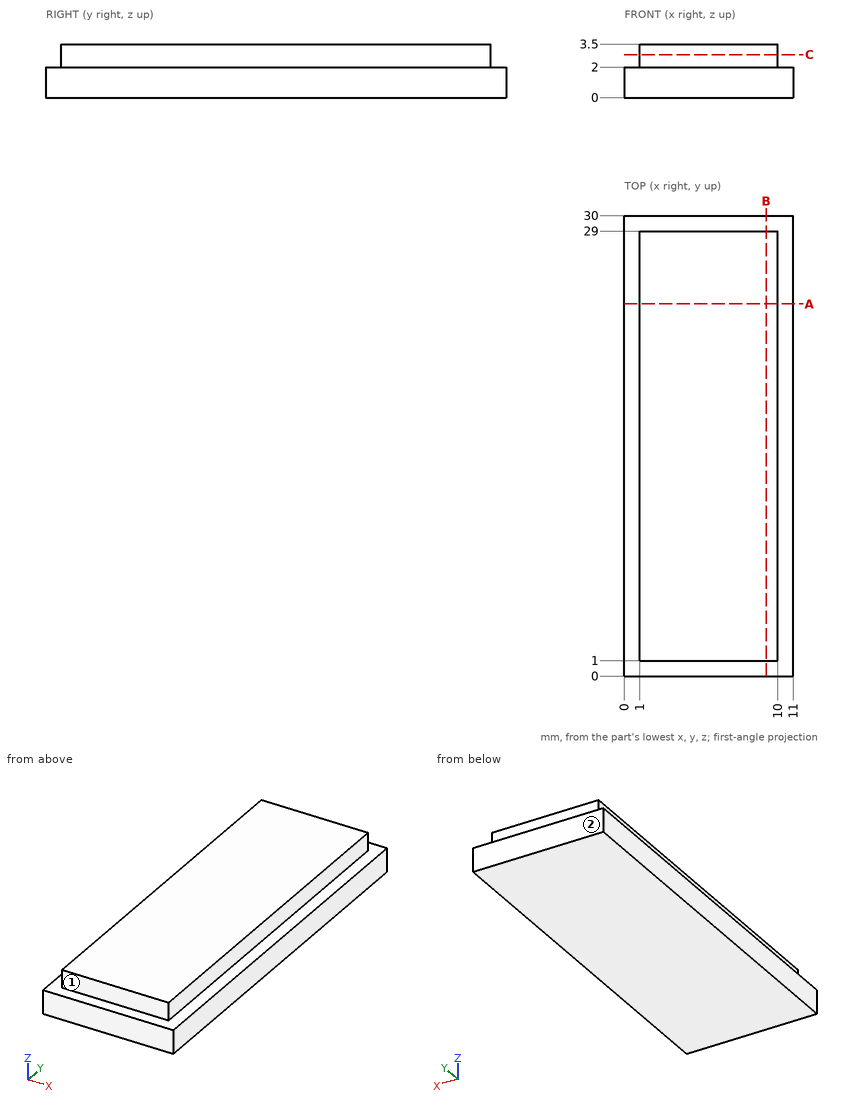
Geometry check sheet. Reference: drawing and pictorial views, mm from the part's lowest x, y, z. A direction names the side the tool comes from. Coordinates: 2 decimals unless noted, no trailing zeros. Loops run counter-clockwise (first coordinate to the right, second up) from the corner with the lowest first, then second, coordinate; pieces in that order, holes last.
1) Gauge pin test, flat ends, axial feed: pin 1 (1.2 mm diameter, centred on x = 7.5, z = 3, fed in from -Y); pin 2 (1.6 mm diameter, centred on y = 13.5, z = 3, fed in from -X). Record the tip position at first contact, or that the pin passes through.
2) Sectioned sample at C-C (z = 2.8). Record the boundary of the cut face in (x, y).
3) Material ranges on probe 1 along X at (y, z) = (18.75, 2.95); probe 2 along Z at (x, y) = (0.5, 14.75); probe 3 along Y at (x, z) = (4, 2.3), recorded low to high.
4) Access from +Z, -Z, +X, -X, +Y, -Y to the whole of each face (thin tool, end or side, straight path). Record for the marked faces 1 and 2.
5) Sectioned sample at A-A (y = 24.25). Record the boundary of the cut face in (x, z).
6) Sectioned sample at B-B (x = 9.25). Record the boundary of the cut face in (y, z).
Check sheet entries:
1. pin 1: stops at y = 1
1. pin 2: stops at x = 1
2. outline: (1, 1) - (10, 1) - (10, 29) - (1, 29) - close
3. probe 1: x = 1 to 10
3. probe 2: z = 0 to 2
3. probe 3: y = 1 to 29
4. face 1: +Z, +X, -X, -Y
4. face 2: +Z, -Z, +X, -X, +Y
5. outline: (0, 0) - (11, 0) - (11, 2) - (10, 2) - (10, 3.5) - (1, 3.5) - (1, 2) - (0, 2) - close
6. outline: (0, 0) - (30, 0) - (30, 2) - (29, 2) - (29, 3.5) - (1, 3.5) - (1, 2) - (0, 2) - close
